The drawing under review shows one solid part. Ordinate dimensions are in mm from its lowest x, y, z. A direction names the side the tool comes from. Coordinates: 2 decimals unless noted, no trailing zeros. Loops run counter-clockwise (first coordinate to the right, second up) from the corner with the lowest first, then second, coordinate; pieces in that order, holes last. Notation, with made-up numbers: (58.5, -36.5) - (68.5, -36.5) arc R11 ccw to (68.5, -18.5) - close; hole circle Ø4 at (40.25, 22.5). An arc over 180 degrees is marked (long way). Answer as a JSON object with one key per item and string values. Group by question number.
Item 1: Mouldability with a two-part tool opening along X and no side actions: class the marked faces 3, 4 and 5 as released by +X, released by -X, zero draft, split by the parting line, or undercut.
Item 2: Tool access review of the marked faces 1 and 2: name each direction out of +Z, -Z, +X, -X, +Y, -Y from which nothing blocks a thin tool from reaching the whole face with its end or side.
Item 3: We need section C-C (x = 10). Give the boundary of the cut face in (y, z).
Item 4: To check wall thickness, follow line 1 (X direction, y = 8.25, z = 2.25); line 2 (X direction, y = 7.5, z = 1); line 3 (X direction, y = 3.25, z = 4.5). State the ranges of each line that lie inside material, in increasing order.
Item 5: Clearance check with flat-ended pins moving along their axes: pin 1 (1 mm diameter, centred on x = 15.5, y = 4, fed in from +Z); pin 2 (1.5 mm diameter, centred on x = 21, y = 5, fed in from +Z); pin 3 (4 mm diameter, centred on x = 25.5, y = 10.5, fed in from -Z). State where each tip first meets the part, or that it passes through.
Item 6: We need section A-A (y = 6). Give the boundary of the cut face in (x, z), then the cut area to 3 significant figures.
Item 7: We need section D-D (x = 16.5). Give the boundary of the cut face in (y, z), then the cut area to 3 significant figures.
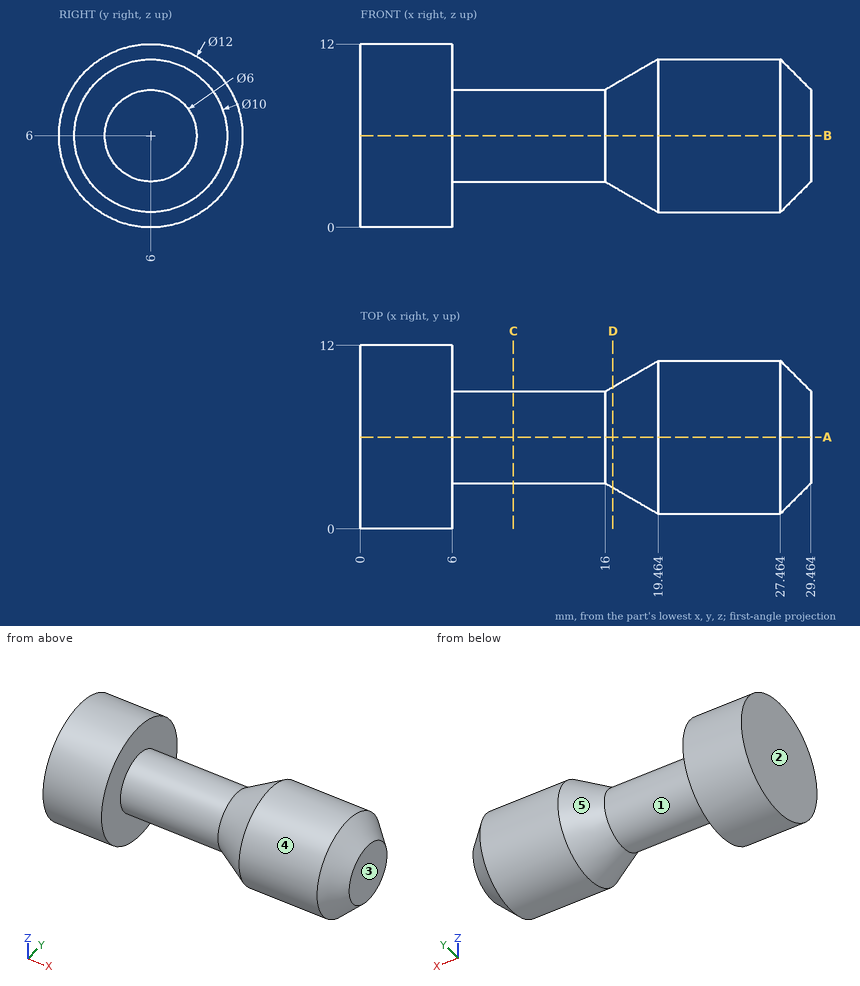
Check sheet entries:
{
 "1": {"face 3": "released by +X", "face 4": "zero draft", "face 5": "undercut"},
 "2": {"face 1": "none", "face 2": "+Z, -Z, -X, +Y, -Y"},
 "3": {"outline": "circle Ø6 at (6, 6)"},
 "4": {"line 1": "x = 0 to 6, 18.38 to 28.09", "line 2": "x = 0 to 6", "line 3": "x = 0 to 6, 16.23 to 29.33"},
 "5": {"pin 1": "stops at z = 8.6", "pin 2": "stops at z = 10.99", "pin 3": "stops at z = 1.67"},
 "6": {"outline": "(0, 0) - (6, 0) - (6, 3) - (16, 3) - (19.46, 1) - (27.46, 1) - (29.46, 3) - (29.46, 9) - (27.46, 11) - (19.46, 11) - (16, 9) - (6, 9) - (6, 12) - (0, 12) - close", "area": "256 mm2"},
 "7": {"outline": "circle Ø6.58 at (6, 6)", "area": "34.0 mm2"}
}
